```python
from build123d import *

# Parameters (mm, degrees)
F0_W     = 90
F0_H     = 20
F0_W_2   = 10
F1_DEPTH = 52
F2_R     = 25.99999
F4_DEPTH = 25
F6_DEPTH = 25


# Not quite as in the source:
# - a fillet or chamfer is up to 0.001 mm smaller than in the source, because OpenCascade refuses the exact size


with BuildPart() as f1:
    # F0 (on Front) → F1 (new body)
    with BuildSketch(Plane.XZ):
        Polygon((-45.2548339959, 45.2548339959), (0, 0), (20, 0), (20, 20), (8.2842712475, 20), (-31.1126983722, 59.3969696197), align=None)
        with Locations((65, 10)):
            Rectangle(F0_W, F0_H)
        Polygon((-59.3969696197, 59.3969696197), (-45.2548339959, 45.2548339959), (-31.1126983722, 59.3969696197), (-45.2548339959, 73.5391052434), align=None)
        with Locations((115, 10)):
            Rectangle(F0_W_2, F0_H)
        Polygon((-70.7106781187, 70.7106781187), (-59.3969696197, 59.3969696197), (-45.2548339959, 73.5391052434), (-56.5685424949, 84.8528137424), align=None)
    extrude(amount=F1_DEPTH)

    # F2 (radius 26 in the source; OpenCascade refuses exactly that, so slightly less here)
    f2_edges = [f1.edges().sort_by_distance(p)[0] for p in [
        (-63.63961, 0, 77.781746),
        (-63.63961, -52, 77.781746),
    ]]
    fillet(f2_edges, radius=F2_R)

    # F3 (on face) → F4 (cut)
    with BuildSketch(Plane(origin=(14.1421356237, 0, 14.1421356237), x_dir=(0.7071067812, 0, -0.7071067812), z_dir=(0.7071067812, 0, 0.7071067812))):
        with BuildLine():
            ThreePointArc((-84, -26), (-74, -36), (-64, -26))
            ThreePointArc((-64, -26), (-74, -16), (-84, -26))
        make_face()
    extrude(amount=-F4_DEPTH, mode=Mode.SUBTRACT)

    # F5 (on face) → F6 (cut)
    with BuildSketch(Plane.XY.offset(20)):
        with BuildLine():
            Line((100, -16), (30, -16))
            ThreePointArc((30, -16), (22.9289321881, -18.9289321881), (20, -26))
            ThreePointArc((20, -26), (22.9289321881, -33.0710678119), (30, -36))
            Line((30, -36), (100, -36))
            ThreePointArc((100, -36), (107.0710678119, -33.0710678119), (110, -26))
            ThreePointArc((110, -26), (107.0710678119, -18.9289321881), (100, -16))
        make_face()
    extrude(amount=-F6_DEPTH, mode=Mode.SUBTRACT)


solid = f1.part
```
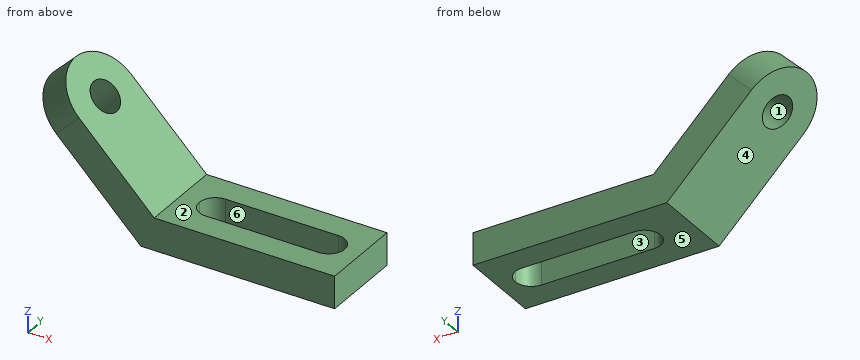
Here's how the part is built. I have some questions about the finished solid (model axes, mm). Face numbers are marked on the shaded views. A direction names the side the tool comes from. Round coordinates to 2 decimals unless told otherwise and drop trailing zeros. Loops run counter-clockwise (first coordinate to the right, second up) from the corner with the lowest first, then second, coordinate; pieces in that order, holes last.
1. Suppose I cut it at C-C, the plane y = -19. Please give me the cut outline in (x, z).
Answers:
outline: (-70.03, 70.03) - (-57.38, 57.38) - (-43.23, 71.52) - (-55.89, 84.17) - close; (-47.28, 47.28) - (0, 0) - (22.86, 0) - (22.86, 20) - (8.28, 20) - (-33.13, 61.42) - close; (107.14, 0) - (120, 0) - (120, 20) - (107.14, 20) - close
2. For the marked faces 5 and 6, which set-ups out of +Z, -Z, +X, -X, +Y, -Y let a thin tool reach every point of the face, with its end or its side?
Answers:
face 5: -Z, +X, -X, +Y, -Y
face 6: +Z, -Z
3. Will these pins go through, and if not, where does the flat tip stop? pin 1 (12 mm diameter, centred on x = 28, y = -14, fed in from +Z); pin 2 (8 mm diameter, centred on x = -28, y = -46, fed in from -Z); pin 3 (4 mm diameter, centred on y = -24.5, z = 67, fed in from -X); pin 4 (12 mm diameter, centred on x = 44, y = -28, fed in from -Z).
Answers:
pin 1: stops at z = 20
pin 2: stops at z = 24
pin 3: stops at x = -69
pin 4: passes through
4. Suppose I cut it at B-B, the plane z = 5. Please give me the cut outline in (x, y).
Answers:
outline: (-5, -52) - (120, -52) - (120, 0) - (-5, 0) - close; hole (30, -36) - (100, -36) arc R10 ccw to (100, -16) - (30, -16) arc R10 ccw to start
5. If I drill on probe 1 along Y at (x, z) = (64, 4); probe 2 along Z at (x, y) = (11.5, -48); probe 3 along X at (y, z) = (-27.5, 44), over which ranges is the centre line in solid material (lowest first)?
Answers:
probe 1: y = -52 to -36, -16 to 0
probe 2: z = 0 to 20
probe 3: x = -44 to -15.72
6. Suppose I cut it at D-D, the plane y = -43.5. Please give me the cut outline in (x, z), and give its area (3 significant figures).
Answers:
outline: (-65.92, 65.92) - (0, 0) - (120, 0) - (120, 20) - (8.28, 20) - (-51.78, 80.06) - close
area: 4,100 mm2
7. Thinking about a two-plate mould opening in X: for the marked faces 1, 2, 3 and 4, which applies, released by +X, released by -X, zero draft, split by the parting line, or undercut?
Answers:
face 1: undercut
face 2: zero draft
face 3: undercut
face 4: released by -X
8. Suppose I cut it at A-A, the plane x = 39. Please give me the cut outline in (y, z), and give its area (3 significant figures).
Answers:
outline: (-52, 0) - (-36, 0) - (-36, 20) - (-52, 20) - close; (-16, 0) - (0, 0) - (0, 20) - (-16, 20) - close
area: 640 mm2
